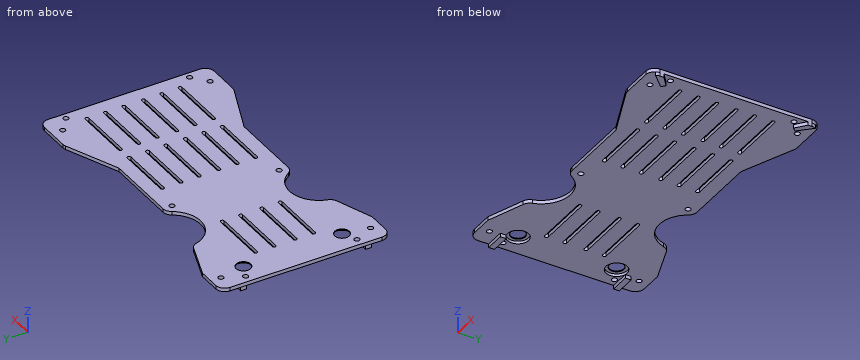
```python
from build123d import *

# Parameters (mm, degrees)
F0_R     = 1.5
F0_R_2   = 4.064442
F1_DEPTH = 2
F2_W     = 10.996489
F2_H     = 3.251471
F3_DEPTH = 2
F4_R     = 5.902111
F5_DEPTH = 1.5


with BuildPart() as f1:
    # F0 (on Top) → F1 (new body)
    with BuildSketch(Plane.XY):
        with BuildLine():
            ThreePointArc((0, 42.5), (-1.464466, 46.035534), (-5, 47.5))
            Line((-5, 47.5), (-22.221084, 47.5))
            ThreePointArc((-22.221084, 47.5), (-23.18507, 47.406193), (-24.112885, 47.128292))
            Line((-24.112885, 47.128292), (-53.784762, 35))
            Line((-53.784762, 35), (-94.883973, 35))
            ThreePointArc((-94.883973, 35), (-97.317732, 34.367701), (-99.135947, 32.630726))
            ThreePointArc((-99.135947, 32.630726), (-115.303652, 25.021468), (-128.810321, 36.720415))
            ThreePointArc((-128.810321, 36.720415), (-129.96409, 38.753765), (-131.916134, 40.040317))
            Line((-131.916134, 40.040317), (-152.559489, 47.5))
            Line((-152.559489, 47.5), (-165, 47.5))
            ThreePointArc((-165, 47.5), (-168.535534, 46.035534), (-170, 42.5))
            Line((-170, 42.5), (-170, 35))
            Line((-170, 35), (-170, 0))
            Line((-170, 0), (-170, -35))
            Line((-170, -35), (-170, -42.5))
            ThreePointArc((-170, -42.5), (-168.535534, -46.035534), (-165, -47.5))
            Line((-165, -47.5), (-152.559489, -47.5))
            Line((-152.559489, -47.5), (-131.916134, -40.040317))
            ThreePointArc((-131.916134, -40.040317), (-129.96409, -38.753765), (-128.810321, -36.720415))
            ThreePointArc((-128.810321, -36.720415), (-115.303652, -25.021468), (-99.135947, -32.630726))
            ThreePointArc((-99.135947, -32.630726), (-97.317732, -34.367701), (-94.883973, -35))
            Line((-94.883973, -35), (-53.784762, -35))
            Line((-53.784762, -35), (-24.112885, -47.128292))
            ThreePointArc((-24.112885, -47.128292), (-23.18507, -47.406193), (-22.221084, -47.5))
            Line((-22.221084, -47.5), (-5, -47.5))
            ThreePointArc((-5, -47.5), (-1.464466, -46.035534), (0, -42.5))
            Line((0, -42.5), (0, -35))
            Line((0, -35), (0, 0))
            Line((0, 0), (0, 35))
            Line((0, 35), (0, 42.5))
        make_face()
        with Locations((-160.42681, -41.874927)):
            Circle(F0_R, mode=Mode.SUBTRACT)
        with Locations((-165.596247, -31.161871)):
            Circle(F0_R, mode=Mode.SUBTRACT)
        with Locations((-157.563224, -27.604574)):
            Circle(F0_R_2, mode=Mode.SUBTRACT)
        with Locations((-94.883973, -30)):
            Circle(F0_R, mode=Mode.SUBTRACT)
        with BuildLine():
            Line((-149.953485, -15.195275), (-118.92181, -15.195275))
            ThreePointArc((-118.92181, -15.195275), (-117.92181, -16.195275), (-118.92181, -17.195275))
            Line((-118.92181, -17.195275), (-149.953485, -17.195275))
            ThreePointArc((-149.953485, -17.195275), (-150.953485, -16.195275), (-149.953485, -15.195275))
        make_face(mode=Mode.SUBTRACT)
        with BuildLine():
            ThreePointArc((-118.92181, -4.895275), (-117.92181, -5.895275), (-118.92181, -6.895275))
            Line((-118.92181, -6.895275), (-149.953485, -6.895275))
            ThreePointArc((-149.953485, -6.895275), (-150.953485, -5.895275), (-149.953485, -4.895275))
            Line((-149.953485, -4.895275), (-118.92181, -4.895275))
        make_face(mode=Mode.SUBTRACT)
        with BuildLine():
            ThreePointArc((-48.304251, -25.082428), (-47.304251, -26.082428), (-48.304251, -27.082428))
            Line((-48.304251, -27.082428), (-79.335926, -27.082428))
            ThreePointArc((-79.335926, -27.082428), (-80.335926, -26.082428), (-79.335926, -25.082428))
            Line((-79.335926, -25.082428), (-48.304251, -25.082428))
        make_face(mode=Mode.SUBTRACT)
        with Locations((-11.601751, -41.25)):
            Circle(F0_R, mode=Mode.SUBTRACT)
        with BuildLine():
            Line((-40.035926, -25.082428), (-9.004251, -25.082428))
            ThreePointArc((-9.004251, -25.082428), (-8.004251, -26.082428), (-9.004251, -27.082428))
            Line((-9.004251, -27.082428), (-40.035926, -27.082428))
            ThreePointArc((-40.035926, -27.082428), (-41.035926, -26.082428), (-40.035926, -25.082428))
        make_face(mode=Mode.SUBTRACT)
        with Locations((-3.568025, -34.615397)):
            Circle(F0_R, mode=Mode.SUBTRACT)
        with BuildLine():
            Line((-79.335926, -14.782428), (-48.304251, -14.782428))
            ThreePointArc((-48.304251, -14.782428), (-47.304251, -15.782428), (-48.304251, -16.782428))
            Line((-48.304251, -16.782428), (-79.335926, -16.782428))
            ThreePointArc((-79.335926, -16.782428), (-80.335926, -15.782428), (-79.335926, -14.782428))
        make_face(mode=Mode.SUBTRACT)
        with BuildLine():
            ThreePointArc((-48.304251, -4.482428), (-47.304251, -5.482428), (-48.304251, -6.482428))
            Line((-48.304251, -6.482428), (-79.335926, -6.482428))
            ThreePointArc((-79.335926, -6.482428), (-80.335926, -5.482428), (-79.335926, -4.482428))
            Line((-79.335926, -4.482428), (-48.304251, -4.482428))
        make_face(mode=Mode.SUBTRACT)
        with BuildLine():
            Line((-40.035926, -14.782428), (-9.004251, -14.782428))
            ThreePointArc((-9.004251, -14.782428), (-8.004251, -15.782428), (-9.004251, -16.782428))
            Line((-9.004251, -16.782428), (-40.035926, -16.782428))
            ThreePointArc((-40.035926, -16.782428), (-41.035926, -15.782428), (-40.035926, -14.782428))
        make_face(mode=Mode.SUBTRACT)
        with BuildLine():
            ThreePointArc((-9.004251, -4.482428), (-8.004251, -5.482428), (-9.004251, -6.482428))
            Line((-9.004251, -6.482428), (-40.035926, -6.482428))
            ThreePointArc((-40.035926, -6.482428), (-41.035926, -5.482428), (-40.035926, -4.482428))
            Line((-40.035926, -4.482428), (-9.004251, -4.482428))
        make_face(mode=Mode.SUBTRACT)
        with BuildLine():
            Line((-149.953485, 6.895275), (-118.92181, 6.895275))
            ThreePointArc((-118.92181, 6.895275), (-117.92181, 5.895275), (-118.92181, 4.895275))
            Line((-118.92181, 4.895275), (-149.953485, 4.895275))
            ThreePointArc((-149.953485, 4.895275), (-150.953485, 5.895275), (-149.953485, 6.895275))
        make_face(mode=Mode.SUBTRACT)
        with BuildLine():
            Line((-149.953485, 17.195275), (-118.92181, 17.195275))
            ThreePointArc((-118.92181, 17.195275), (-117.92181, 16.195275), (-118.92181, 15.195275))
            Line((-118.92181, 15.195275), (-149.953485, 15.195275))
            ThreePointArc((-149.953485, 15.195275), (-150.953485, 16.195275), (-149.953485, 17.195275))
        make_face(mode=Mode.SUBTRACT)
        with Locations((-157.563224, 27.604574)):
            Circle(F0_R_2, mode=Mode.SUBTRACT)
        with Locations((-165.596247, 31.161871)):
            Circle(F0_R, mode=Mode.SUBTRACT)
        with Locations((-160.42681, 41.874927)):
            Circle(F0_R, mode=Mode.SUBTRACT)
        with Locations((-94.883973, 30)):
            Circle(F0_R, mode=Mode.SUBTRACT)
        with BuildLine():
            Line((-79.335926, 6.482428), (-48.304251, 6.482428))
            ThreePointArc((-48.304251, 6.482428), (-47.304251, 5.482428), (-48.304251, 4.482428))
            Line((-48.304251, 4.482428), (-79.335926, 4.482428))
            ThreePointArc((-79.335926, 4.482428), (-80.335926, 5.482428), (-79.335926, 6.482428))
        make_face(mode=Mode.SUBTRACT)
        with BuildLine():
            Line((-79.335926, 16.782428), (-48.304251, 16.782428))
            ThreePointArc((-48.304251, 16.782428), (-47.304251, 15.782428), (-48.304251, 14.782428))
            Line((-48.304251, 14.782428), (-79.335926, 14.782428))
            ThreePointArc((-79.335926, 14.782428), (-80.335926, 15.782428), (-79.335926, 16.782428))
        make_face(mode=Mode.SUBTRACT)
        with BuildLine():
            Line((-40.035926, 6.482428), (-9.004251, 6.482428))
            ThreePointArc((-9.004251, 6.482428), (-8.004251, 5.482428), (-9.004251, 4.482428))
            Line((-9.004251, 4.482428), (-40.035926, 4.482428))
            ThreePointArc((-40.035926, 4.482428), (-41.035926, 5.482428), (-40.035926, 6.482428))
        make_face(mode=Mode.SUBTRACT)
        with BuildLine():
            Line((-40.035926, 16.782428), (-9.004251, 16.782428))
            ThreePointArc((-9.004251, 16.782428), (-8.004251, 15.782428), (-9.004251, 14.782428))
            Line((-9.004251, 14.782428), (-40.035926, 14.782428))
            ThreePointArc((-40.035926, 14.782428), (-41.035926, 15.782428), (-40.035926, 16.782428))
        make_face(mode=Mode.SUBTRACT)
        with BuildLine():
            Line((-79.335926, 27.082428), (-48.304251, 27.082428))
            ThreePointArc((-48.304251, 27.082428), (-47.304251, 26.082428), (-48.304251, 25.082428))
            Line((-48.304251, 25.082428), (-79.335926, 25.082428))
            ThreePointArc((-79.335926, 25.082428), (-80.335926, 26.082428), (-79.335926, 27.082428))
        make_face(mode=Mode.SUBTRACT)
        with BuildLine():
            Line((-40.035926, 27.082428), (-9.004251, 27.082428))
            ThreePointArc((-9.004251, 27.082428), (-8.004251, 26.082428), (-9.004251, 25.082428))
            Line((-9.004251, 25.082428), (-40.035926, 25.082428))
            ThreePointArc((-40.035926, 25.082428), (-41.035926, 26.082428), (-40.035926, 27.082428))
        make_face(mode=Mode.SUBTRACT)
        with Locations((-3.568025, 34.615397)):
            Circle(F0_R, mode=Mode.SUBTRACT)
        with Locations((-11.601751, 41.25)):
            Circle(F0_R, mode=Mode.SUBTRACT)
    extrude(amount=F1_DEPTH)

    # F2 (on face) → F3 (join)
    with BuildSketch(Plane(origin=(0, 0, 0), x_dir=(1, 0, 0), z_dir=(0, 0, -1))):
        with Locations((-164.501756, 34.962811)):
            Rectangle(F2_W, F2_H)
        with BuildLine():
            Line((-0.535832, 44.751933), (-7.695868, 37.591897))
            Line((-7.695868, 37.591897), (-5.774221, 35.670251))
            Line((-5.774221, 35.670251), (0, 40.31283))
            Line((0, 40.31283), (0, 42.5))
            ThreePointArc((0, 42.5), (-0.135802, 43.657402), (-0.535832, 44.751933))
        make_face()
        with BuildLine():
            Line((0, -42.5), (0, -40.31283))
            Line((0, -40.31283), (-5.774221, -35.670251))
            Line((-5.774221, -35.670251), (-7.695868, -37.591897))
            Line((-7.695868, -37.591897), (-0.535832, -44.751933))
            ThreePointArc((-0.535832, -44.751933), (-0.135802, -43.657402), (0, -42.5))
        make_face()
        with Locations((-164.501756, -34.962811)):
            Rectangle(F2_W, F2_H)
    extrude(amount=F3_DEPTH)

    # F4 (on face) → F5 (cut)
    with BuildSketch(Plane(origin=(0, 0, 0), x_dir=(1, 0, 0), z_dir=(0, 0, -1))):
        with Locations((-157.563224, 27.604574)):
            Circle(F4_R)
        with Locations((-157.563224, -27.604574)):
            Circle(F4_R)
    extrude(amount=-F5_DEPTH, mode=Mode.SUBTRACT)


solid = f1.part
```
Work out the finished part from the listing and answer in its coordinate system (mm). Coordinates: 2 decimals unless noted, no trailing zeros. Loops run counter-clockwise (first coordinate to the right, second up) from the corner with the lowest first, then second, coordinate; pieces in that order, holes last. Notation, with made-up numbers: M 65.5,32.25 L 81.5,32.25 A22 cw 81.5,59.25 Z; hole C -35.75,20 d9. An arc over 180 degrees is marked long. Use CSV: the item, a comma, the result in double quotes. Start each with the question number.
(1) Find section A-A, the plane x = -60.5. Give the vertices of the cut face in (y, z), then the cut area to 3 significant figures.
(2) Find section B-B, the plane z = -1.35. Give the vertices of the cut face in (x, y).
(3) Find section D-D, the plane y = -20. Give the vertices of the cut face in (x, z), then the cut area to 3 significant figures.
(4) Consider line 1 (X direction, y = -16, z = 1.7); line 2 (Y direction, x = -158.5, z = 1.3); line 3 (Z direction, x = -13, y = 12). Determine where each line is inside the solid, lowest interval first.
(5) Given pin 1 Ø1.6 at (y, z) = (-35.5, -1) entering from +X; pin 2 Ø2 at (x, z) = (-163, -0.5) entering from +Y; pin 3 Ø1 at (x, z) = (-128.5, 0.5) entering from +Y; pin 4 Ø7 at (x, y) = (-157.56, -27.6) entering from -Z, each flat-ended and moving along its own axis, determine where each tip first touches the part or whether it passes through.
(6) Find section C-C, the plane x = -123. Give the vertices of the cut face in (y, z).
Recorded:
1,outline,"M -35,0 L -27.08,0 L -27.08,2 L -35,2 Z; M -25.08,0 L -16.78,0 L -16.78,2 L -25.08,2 Z; M -14.78,0 L -6.48,0 L -6.48,2 L -14.78,2 Z; M -4.48,0 L 4.48,0 L 4.48,2 L -4.48,2 Z; M 6.48,0 L 14.78,0 L 14.78,2 L 6.48,2 Z; M 16.78,0 L 25.08,0 L 25.08,2 L 16.78,2 Z; M 27.08,0 L 35,0 L 35,2 L 27.08,2 Z"
1,area,"116 mm^2"
2,outline,"M -170,-36.59 L -159,-36.59 L -159,-33.34 L -170,-33.34 Z; M -170,33.34 L -159,33.34 L -159,36.59 L -170,36.59 Z; M -7.7,-37.59 L -0.54,-44.75 A5 ccw 0,-42.5 L 0,-40.31 L -5.77,-35.67 Z; M -7.7,37.59 L -5.77,35.67 L 0,40.31 L 0,42.5 A5 ccw -0.54,44.75 Z"
3,outline,"M -170,0 L 0,0 L 0,2 L -170,2 Z"
3,area,"340 mm^2"
4,line 1,"x = -170 to -150.93, -117.94 to -80.31, -47.33 to -41.01, -8.03 to 0"
4,line 2,"y = -47.5 to -33.43, -21.78 to 21.78, 33.43 to 47.5"
4,line 3,"z = 0 to 2"
5,pin 1,"stops at x = -4.99"
5,pin 2,"stops at y = 47.5"
5,pin 3,"stops at y = 37.26"
5,pin 4,"passes through"
6,outline,"M -28.22,0 L -17.2,0 L -17.2,2 L -28.22,2 Z; M -15.2,0 L -6.9,0 L -6.9,2 L -15.2,2 Z; M -4.9,0 L 4.9,0 L 4.9,2 L -4.9,2 Z; M 6.9,0 L 15.2,0 L 15.2,2 L 6.9,2 Z; M 17.2,0 L 28.22,0 L 28.22,2 L 17.2,2 Z"
